Geometry check sheet. Reference: the model listing, model coordinates, mm. A direction names the side the tool comes from. Round coordinates to 2 decimals unless told otherwise and drop trailing zeros. Loops run counter-clockwise (first coordinate to the right, second up) from the corner with the lowest first, then second, coordinate; pieces in that order, holes last. Notation, with made-up numbers: (-33, -2.5) - (-19, -2.5) arc R25 cw to (-19, 24.5) - close; hole circle Ø9 at (-5.75, 41.5). An arc over 180 degrees is marked (long way). Answer as CSV lines item,"result". Start each with the question number.
1) Access from +Z, -Z, +X, -X, +Y, -Y to the whole of each face (thin tool, end or side, straight path). Record for faces 5 (the flat face through (54, -40, 81)), 6 (the flat face through (20, -20, 44)), 7 (the flat face through (34, -18, 0)), 8 (the flat face through (70, -18, 52)), 9 (the flat face through (46, -39, 45)).
2) Cross-section at C-C on z = 26. Record the boundary of the cut face in (x, y).
3) Cross-section at D-D on x = 56.5. Record the boundary of the cut face in (y, z), and give its area (3 significant figures).
4) Cross-section at A-A on x = 22. Record the boundary of the cut face in (y, z).
5) Cross-section at B-B on y = -40. Record the boundary of the cut face in (x, z).
6) Draft check along Z on faces 1 (the flat face through (68, -30, 103)), 2 (the flat face through (46, -30, 69)), 3 (the flat face through (44, -39, 57)), 4 (the flat face through (46, -30, 23)). Enter one of: released by +Z, released by -Z, zero draft, split by the parting line, or undercut.
7) Depth check by flat-ended pin: P1, Ø3, axis at x = 19, z = 27, coming from the -Y side; P2, Ø6, axis at y = -16.5, z = 22.5, coming from the -X side; P3, Ø4, axis at y = -11, z = 54.5, coming from the +X side; P4, Ø1, axis at x = 35.5, y = -43.5, coming from the +Z side. Enter the tip coordinate at first touch or a pass-through.
8) Thickness scan on line 1 along X through (y, z) = (-13.5, 18); line 2 along Y through (x, z) = (22.5, 60.5); line 3 along Z through (x, y) = (50.5, -33). Record the ranges inside material, lowest first.
Solid Edge part; units mm, degrees
sketch "Sketch1" plane through (0, 0, 0) normal (0, -1, 0) x (1, 0, 0)
  line L0 (90, 45) -> (0, 45)
  line L1 (0, 45) -> (0, 0)
  line L2 (0, 0) -> (90, 0)
  line L3 (90, 0) -> (90, 45)
extrude "Protrusion1" add sketch "Sketch1" along normal blind 30
sketch "Sketch2" plane through (0, 0, 0) normal (0, -1, 0) x (1, 0, 0)
  line L0 (0, 57) -> (90, 57)
  line L1 (90, 57) -> (90, 45)
  line L2 (90, 45) -> (0, 45)
  line L3 (0, 45) -> (0, 57)
extrude "ExtrudedProtrusion_5" add sketch "Sketch2" along normal blind 48
sketch "Sketch3" plane through (0, 0, 0) normal (0, -1, 0) x (1, 0, 0)
  line L0 (90, 81) -> (17.5, 81)
  line L1 (0, 67) -> (17.5, 81)
  line L2 (0, 57) -> (0, 67)
  line L3 (0, 57) -> (90, 57)
  line L4 (90, 67) -> (90, 57)
  line L5 (90, 67) -> (90, 81)
extrude "ExtrudedProtrusion_6" add sketch "Sketch3" along normal blind 30
sketch "Sketch4" plane through (0, 0, 0) normal (0, -1, 0) x (1, 0, 0)
  line L0 (45, 103) -> (17.5, 81)
  line L1 (90, 81) -> (17.5, 81)
  line L2 (90, 81) -> (90, 103)
  line L3 (90, 103) -> (45, 103)
extrude "ExtrudedProtrusion_7" add sketch "Sketch4" along normal blind 50
sketch "Sketch5" plane through (67.5, -25, 103) normal (0, 0, 1) x (1, 0, 0)
  line L0 (22.5, 7) -> (-17.5, 7)
  line L1 (-17.5, 7) -> (-17.5, 25)
  line L2 (-17.5, 25) -> (22.5, 25)
  line L3 (22.5, 25) -> (22.5, 7)
extrude "Cutout1" cut sketch "Sketch5" against normal up to next
sketch "Sketch6" plane through (67.5, -25, 103) normal (0, 0, 1) x (1, 0, 0)
  line L0 (-51.8826, 17) -> (-51.8826, 5)
  line L1 (-51.8826, 5) -> (-42.5122, 5)
  line L2 (-42.5122, 5) -> (-42.5122, 17)
  line L3 (-42.5122, 17) -> (-51.8826, 17)
extrude "Cutout2" cut sketch "Sketch6" against normal up to next
Answer block:
1,face 5,"+X, -X, -Y"
1,face 6,"+Z, -Z"
1,face 7,"-Z, +X, -X, +Y, -Y"
1,face 8,"+Z, -Z, +X, +Y"
1,face 9,"-Z, +X, -X, -Y"
2,outline,"(0, -30) - (90, -30) - (90, -18) - (50, -18) - (50, 0) - (0, 0) - close; hole (15.62, -20) - (24.99, -20) - (24.99, -8) - (15.62, -8) - close"
3,outline,"(-50, 81) - (-30, 81) - (-30, 57) - (-48, 57) - (-48, 45) - (-30, 45) - (-30, 0) - (-18, 0) - (-18, 103) - (-50, 103) - close"
3,area,"1,890 mm^2"
4,outline,"(-50, 81) - (-30, 81) - (-30, 57) - (-48, 57) - (-48, 45) - (-30, 45) - (-30, 0) - (-20, 0) - (-20, 84.6) - (-50, 84.6) - close; (-8, 0) - (0, 0) - (0, 84.6) - (-8, 84.6) - close"
5,outline,"(0, 45) - (90, 45) - (90, 57) - (0, 57) - close; (17.5, 81) - (90, 81) - (90, 103) - (45, 103) - close"
6,face 1,"released by +Z"
6,face 2,"undercut"
6,face 3,"undercut"
6,face 4,"zero draft"
7,P1,"stops at y = -30"
7,P2,"stops at x = 0"
7,P3,"stops at x = 50"
7,P4,"stops at z = 95.8"
8,line 1,"x = 0 to 15.62, 24.99 to 50"
8,line 2,"y = -30 to -20, -8 to 0"
8,line 3,"z = 45 to 57, 81 to 103"
